Verification items for the finished model (mm, model axes). Give positions to 0.01 mm unless a question says otherwise; leave off trailing zeros. Write each loop counter-clockwise with the first axis right and the second up, starting at its lowest first coordinate (ties: lowest second). Pieces come first, ordered by that corner, then holes. Notation, with made-up numbers: (79, -25) -> (133, -25) arc R20 cw to (133, 11) -> close; hole circle Ø5 at (78, 29.25). An arc over 180 degrees is marked (long way). Use one line per item in the form item = value. Start each with the question number.
(1) Section check A-A, the plane y = -365. Record the cut outline in (x, z).
(2) Scan lines: L1, parallel to Y at x = -4, z = -3; L2, parallel to Z at x = -1.25, y = -349; L3, parallel to Y at x = -1.25, z = -40. Record each from-to range of solid material in increasing order.
(3) Depth check by flat-ended pin: pin 1 Ø3 at (x, y) = (-1.5, -378) entering from +Z. Enter the tip coordinate at first touch or a pass-through.
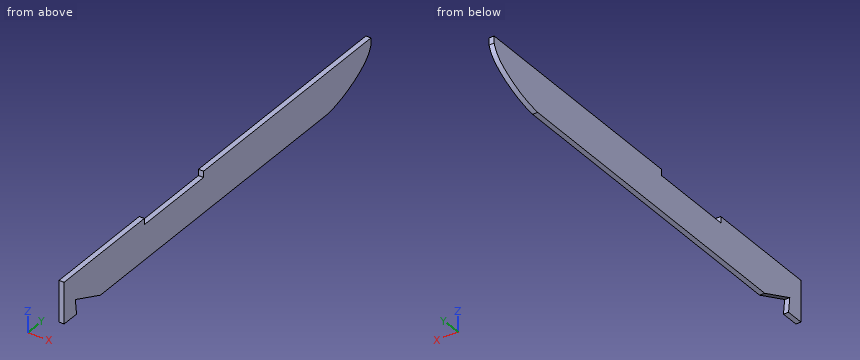
from build123d import *

# Parameters (mm, degrees)
F0_W     = 6.35
F0_H     = 50.8
F1_DEPTH = 558.8
F3_DEPTH = 304.8
F4_W     = 107.95
F4_H     = 7.62
F5_DEPTH = 304.8
F7_DEPTH = 25.4


with BuildPart() as f1:
    # F0 (on Front) → F1 (new body)
    with BuildSketch(Plane.XZ):
        with Locations((-3.175, -25.4)):
            Rectangle(F0_W, F0_H)
    extrude(amount=F1_DEPTH)

    # F2 (on face) → F3 (cut)
    with BuildSketch(Plane.YZ):
        Polygon((-538.3797883987, -31.9133784294), (-536.1839532852, -50.8), (-492.8166270256, -50.8), align=None)
    extrude(amount=-F3_DEPTH, mode=Mode.SUBTRACT)

    # F4 (on face) → F5 (cut)
    with BuildSketch(Plane.YZ):
        with Locations((-358.775, -3.81)):
            Rectangle(F4_W, F4_H)
    extrude(amount=-F5_DEPTH, mode=Mode.SUBTRACT)

    # F6 (on face) → F7 (cut)
    with BuildSketch(Plane.YZ):
        with BuildLine():
            Line((0, -50.8), (0, -8.7046129629))
            add(Edge.make_bspline(
                [(0, -8.7046129629), (-2.2023392611, -14.2512334073), (-9.3405414865, -27.9675195006), (-51.0574173798, -47.8762926406), (-79.2421847582, -50.8)],
                knots=[0, 0, 0, 0, 0.3372731327, 1, 1, 1, 1], degree=3))
            Line((-79.2421847582, -50.8), (0, -50.8))
        make_face()
    extrude(amount=-F7_DEPTH, mode=Mode.SUBTRACT)


solid = f1.part
Completed:
q1.outline = (-6.35, -50.8) -> (0, -50.8) -> (0, -7.62) -> (-6.35, -7.62) -> close
q2.L1 = -558.8 to -412.75, -304.8 to 0
q2.L2 = -50.8 to -7.62
q2.L3 = -558.8 to -537.44, -518.87 to -38.4
q3.pin_1 = -7.62
